The model under review builds one solid part; all positions refer to its coordinate system, in mm. Face numbers are marked on the shaded views. A direction names the side the tool comes from. Give positions to 0.01 mm unless a question says otherwise; leave off trailing zeros. Write each loop counter-clockwise with the first axis right and the second up, starting at its lowest first coordinate (ties: lowest second). Pieces come first, ordered by that corner, then holes. Notation, with made-up numbers: (49, 34.25) - (107, 34.25) arc R29 ccw to (107, 56.25) - close; hole circle Ø11 at (77, -28). An arc over 180 degrees is marked (long way). Write item = value, one per line.
```python
from build123d import *

# Parameters (mm, degrees)
SKETCH1_W           = 26
SKETCH1_H           = 32
BOSS_EXTRUDE1_DEPTH = 32
SKETCH2_W           = 45
SKETCH2_H           = 40
SKETCH2_H_2         = 19
BOSS_EXTRUDE2_DEPTH = 52
CHAMFER1_SIZE       = 7
SKETCH3_R           = 7
CUT_EXTRUDE1_DEPTH  = 71.569115058
CHAMFER2_SIZE       = 5
SPLIT1_DEPTH        = 45
CUT_EXTRUDE2_DEPTH  = 52
CUT_EXTRUDE7_DEPTH  = 80.555012413
SKETCH8_R           = 41
CUT_EXTRUDE8_DEPTH  = 24
SKETCH9_R           = 5.5
CUT_EXTRUDE9_DEPTH  = 80.555012413


# Read off the part's stored shape, not the designer's step: Split1
with BuildPart() as part:
    # Sketch1 → Boss-Extrude1 (new body)
    with BuildSketch(Plane(origin=(0, 0, 0), x_dir=(0, 0, -1), z_dir=(1, 0, 0))):
        with Locations((-13, 16)):
            Rectangle(SKETCH1_W, SKETCH1_H)
    extrude(amount=-BOSS_EXTRUDE1_DEPTH)

    # Sketch2 → Boss-Extrude2 (add)
    with BuildSketch(Plane(origin=(0, 0, 0), x_dir=(0, 0, -1), z_dir=(1, 0, 0))):
        with Locations((-22.5, 20)):
            Rectangle(SKETCH2_W, SKETCH2_H)
        with Locations((-22.5, -9.5)):
            Rectangle(SKETCH2_W, SKETCH2_H_2)
    extrude(amount=BOSS_EXTRUDE2_DEPTH)

    # Chamfer1
    chamfer1_edges = [part.edges().sort_by_distance(p)[0] for p in [
        (-32, 0, 13),
        (-32, 32, 13),
    ]]
    chamfer(chamfer1_edges, length=CHAMFER1_SIZE)

    # Sketch3 → Cut-Extrude1 (cut, through all)
    with BuildSketch(Plane.XY.offset(26)):
        with Locations((-18, 14)):
            Circle(SKETCH3_R)
    extrude(amount=-CUT_EXTRUDE1_DEPTH, mode=Mode.SUBTRACT)

    # Chamfer2
    chamfer2_edges = [part.edges().sort_by_distance(p)[0] for p in [
        (52, 40, 22.5),
    ]]
    chamfer(chamfer2_edges, length=CHAMFER2_SIZE)

    # Split1 outline → Split1 (cut)
    with BuildSketch(Plane.XY):
        with BuildLine():
            ThreePointArc((2.104042352, 28.455114912), (14.591637328, 30.535902458), (23, 40))
            Line((23, 40), (0, 40))
            Line((0, 40), (0, 32))
            Line((0, 32), (-18, 32))
            Line((-18, 32), (2.104042352, 28.455114912))
        make_face()
    extrude(amount=SPLIT1_DEPTH, mode=Mode.SUBTRACT)

    # Sketch6 → Cut-Extrude2 (cut)
    with BuildSketch(Plane.XY.offset(45)):
        Polygon((52, -19), (52, 16), (23, -19), align=None)
    extrude(amount=-CUT_EXTRUDE2_DEPTH, mode=Mode.SUBTRACT)

    # Sketch7 → Cut-Extrude7 (cut, through all)
    with BuildSketch(Plane.XY.offset(45)):
        with BuildLine():
            ThreePointArc((18.113465426, -19), (12.616803089, -10.198093068), (10.696969697, 0))
            Line((10.696969697, 0), (0, 0))
            Line((0, 0), (0, -19))
            Line((0, -19), (18.113465426, -19))
        make_face()
    extrude(amount=-CUT_EXTRUDE7_DEPTH, mode=Mode.SUBTRACT)

    # Sketch8 → Cut-Extrude8 (cut)
    with BuildSketch(Plane.XY.offset(12)):
        with Locations((52, 43.758742169)):
            Circle(SKETCH8_R)
    extrude(amount=CUT_EXTRUDE8_DEPTH, mode=Mode.SUBTRACT)

    # Sketch9 → Cut-Extrude9 (cut, through all)
    with BuildSketch(Plane.XY.offset(45)):
        with Locations((38, 26)):
            Circle(SKETCH9_R)
    extrude(amount=-CUT_EXTRUDE9_DEPTH, mode=Mode.SUBTRACT)


solid = part.part
```
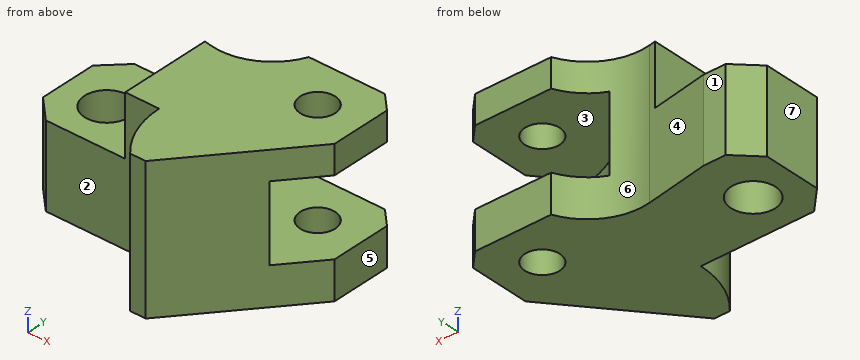
1. Take a section at B-B on x = 38. Give the boundary of the cut face in (y, z).
Findings below:
outline = (-0.9, 0) - (20.5, 0) - (20.5, 12) - (5.22, 12) - (5.22, 36) - (20.5, 36) - (20.5, 45) - (-0.9, 45) - close; (31.5, 0) - (40, 0) - (40, 12) - (31.5, 12) - close; (31.5, 36) - (40, 36) - (40, 45) - (31.5, 45) - close
2. Insertion check: P1, Ø3, axis at x = -9.5, z = 11.5, coming from the -Y side; P2, Ø12, axis at x = -20, y = 1.5, coming from the +Z side; P3, Ø7.5, axis at x = -22.5, z = 15.5, coming from the +Y side. Each pin has a flat end and moves straight along its axis. Give the tip position at first contact, or say it passes through.
Findings below:
P1 = 0
P2 = 26
P3 = 32
3. Draft analysis for pull direction X (two halves, no side actions). For the marked faces 5, 6 and 7, state which applies: +X half, -X half, draft (parallel to the pull), parting line (faces both ways), or undercut.
Findings below:
face_5 = +X half
face_6 = undercut
face_7 = -X half
4. Take a section at C-C on y = 14. Give the boundary of the cut face in (x, z), and give its area (3 significant figures).
Findings below:
outline = (-32, 0) - (-25, 0) - (-25, 26) - (-32, 26) - close; (-11, 0) - (50.34, 0) - (50.34, 12) - (23.8, 12) - (23.8, 36) - (50.34, 36) - (50.34, 45) - (0, 45) - (0, 26) - (-11, 26) - close
area = 2,100 mm²
5. For line 1 (Z direction, x = 47, y = 11); line 2 (Z direction, x = -7.5, y = 2); line 3 (Y direction, x = 38, z = 6), list the stretches that pass through material, from the lowest coordinate up. Write a range as from..to.
Findings below:
line_1 = 0..12, 36..45
line_2 = 0..26
line_3 = -0.9..20.5, 31.5..40
6. Machinability: for the marked faces 1, 2, 3 and 4, which of the approach directions +Z, -Z, +X, -X, +Y, -Y give a long, thin tool a straight path to every point of the face, cutting with its end or side? Answer none if there is none.
Findings below:
face_1 = +Z, -Z, -X, +Y
face_2 = +Z, -Z, -X, -Y
face_3 = +X, +Y
face_4 = +Z, -Z, +Y
7. Take a section at A-A on z = 13. Give the boundary of the cut face in (x, y), and give its area (3 significant figures).
Findings below:
outline = (-32, 7) - (-25, 0) - (10.7, 0) arc R28.05 ccw to (18.11, -19) - (23, -19) - (42.05, 3.99) arc R41 cw to (13.4, 29.93) arc R19 cw to (2.1, 28.46) - (-18, 32) - (-25, 32) - (-32, 25) - close; hole circle Ø14 at (-18, 14)
area = 1,870 mm²
8. Take a section at D-D on z = 28. Give the boundary of the cut face in (x, y), and give its area (3 significant figures).
Findings below:
outline = (0, 0) - (10.7, 0) arc R28.05 ccw to (18.11, -19) - (23, -19) - (42.05, 3.99) arc R41 cw to (13.4, 29.93) arc R19 cw to (2.1, 28.46) - (0, 28.83) - close
area = 1,080 mm²
